Print and shaded views of the part. All mm, measured from the part's lowest x, y and z. Give positions to 0.01 mm unless a question says otherwise; leave off trailing zeros. Loops run counter-clockwise (first coordinate to the right, second up) from the corner with the lowest first, then second, coordinate; pieces in that order, holes last. Notation, with made-up numbers: (29, 76) -> (52, 76) arc R13 cw to (52, 80) -> close; hole circle Ø1 at (55, 3). An arc over 180 degrees is marked (long way). Answer as a JSON object with one key per item and string values. Group by question number.
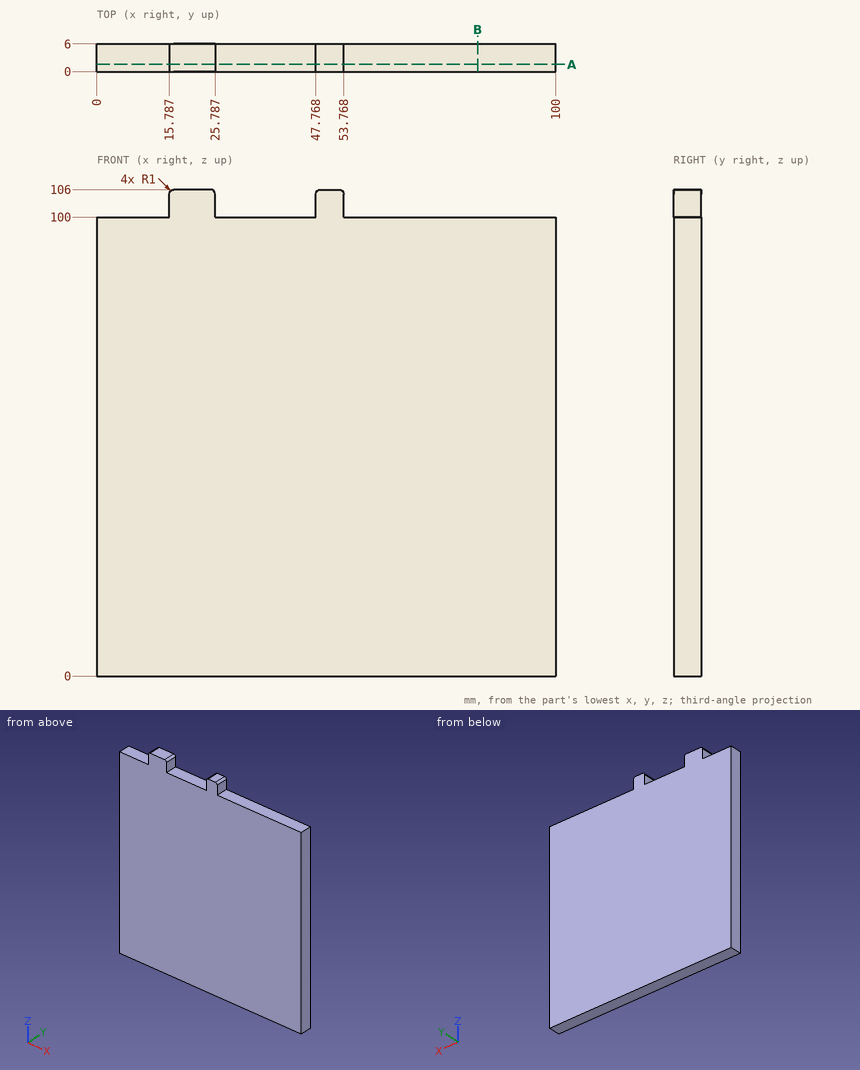
(1) Pin check, flat tips, straight feed: pin 1 (3 mm diameter, centred on x = 74.5, y = 4, fed in from +Z); pin 2 (2.5 mm diameter, centred on y = 3.5, z = 102.5, fed in from -X). Stop position of each tip, or through.
(2) Saw through at A-A on y = 1.55. List the corners of the cut face in (x, z).
(3) Probe line 1 along Z through (x, y) = (9.5, 2.65). List the from-to ranges inside material, lowest first. Write a range as [from, to].
(4) Saw through at B-B on x = 83. List the corners of the cut face in (y, z).
Calculated:
{
 "1": {"pin 1": "stops at z = 100", "pin 2": "stops at x = 15.79"},
 "2": {"outline": "(0, 0) -> (100, 0) -> (100, 100) -> (53.77, 100) -> (53.77, 105) arc R1 ccw to (52.77, 106) -> (48.77, 106) arc R1 ccw to (47.77, 105) -> (47.77, 100) -> (25.79, 100) -> (25.79, 105) arc R1 ccw to (24.79, 106) -> (16.79, 106) arc R1 ccw to (15.79, 105) -> (15.79, 100) -> (0, 100) -> close"},
 "3": {"line 1": "z = [0, 100]"},
 "4": {"outline": "(0, 0) -> (6, 0) -> (6, 100) -> (0, 100) -> close"}
}
